Part model, mm, in its own coordinate system. Face numbers are marked on the shaded views. A direction names the side the tool comes from. Give positions to 0.01 mm unless a question says otherwise; leave off trailing zeros. Write each loop counter-clockwise with the first axis right and the second up, starting at its lowest first coordinate (ties: lowest second). Pieces come first, ordered by that corner, then holes. Notation, with made-up numbers: M 56,75 L 71,75 A15 ccw 71,100 Z; hole C 56,-8 d1. An arc over 180 degrees is marked long. Write item = value, one per line. Start each with the question number.
from build123d import *

# Parameters (mm, degrees)
SKETCH_1_W               = 38
SKETCH_1_H               = 11.5
EXTRUDE_1_DEPTH          = 1.6
EXTRUDE_START            = 1.6
SKETCH_1_3_W             = 38
SKETCH_1_3_H             = 1
SKETCH_1_3_W_2           = 1.5
SKETCH_1_3_H_2           = 11.5
EXTRUDE_2_DEPTH          = 1.5
EXTRUDE_START_2          = 3.1
EXTRUDE_3_DEPTH          = 8.4
SKETCH_2_4_W             = 2.4
SKETCH_2_4_H             = 1.5
EXTRUDE_5_DEPTH          = 3.1
CUT_EXTRUDE_1_DEPTH      = 22.744252114
FILLET_1_R               = 3
EXTRUDE_4_REACH          = 28.684
SKETCH_3_R               = 1.6
CUT_EXTRUDE_2_DEPTH      = 27.684499246
CUT_EXTRUDE_2_DEPTH_BACK = 27.684499246
SKETCH_3_3_R             = 1.7
SKETCH_3_3_W             = 6.5
SKETCH_3_3_H             = 1.7
SKETCH_3_3_W_2           = 3.4
SKETCH_3_3_H_2           = 3.1
FILLET_2_R               = 2.8
FILLET_3_R               = 2.5
FILLET_4_R               = 1
FILLET_5_R               = 0.5
FILLET_6_R               = 2


with BuildPart() as part:
    # 草图1 → 凸台-拉伸1 (new body)
    with BuildSketch(Plane(origin=(0, 0, 0), x_dir=(1, 0, 0), z_dir=(0, 1, 0))):
        Rectangle(SKETCH_1_W, SKETCH_1_H)
    extrude(amount=EXTRUDE_1_DEPTH)

    # 草图1<3> → 凸台-拉伸2 (add)
    with BuildSketch(Plane(origin=(0, 0, 0), x_dir=(1, 0, 0), z_dir=(0, 1, 0)).offset(EXTRUDE_START)):
        with Locations((0, 3.75)):
            Rectangle(SKETCH_1_3_W, SKETCH_1_3_H)
        Rectangle(SKETCH_1_3_W, SKETCH_1_3_H)
        with Locations((0, -3.75)):
            Rectangle(SKETCH_1_3_W, SKETCH_1_3_H)
        with Locations((-11.75, 0)):
            Rectangle(SKETCH_1_3_W_2, SKETCH_1_3_H_2)
        with Locations((11.75, 0)):
            Rectangle(SKETCH_1_3_W_2, SKETCH_1_3_H_2)
    extrude(amount=EXTRUDE_2_DEPTH)

    # 草图2 → 凸台-拉伸3 (add)
    with BuildSketch(Plane(origin=(0, 0, 0), x_dir=(1, 0, 0), z_dir=(0, 1, 0)).offset(EXTRUDE_START_2)):
        Polygon((-3.3, 9.05), (-5.1, 9.05), (-5.1, -2.15), (-7.5, -2.15), (-7.5, -9.15), (-5.5, -9.15), (-5.5, -2.55), (-3.3, -2.55), align=None)
        Polygon((5.1, 9.05), (3.3, 9.05), (3.3, -2.55), (5.5, -2.55), (5.5, -9.15), (7.5, -9.15), (7.5, -2.15), (5.1, -2.15), align=None)
    extrude(amount=-EXTRUDE_3_DEPTH)

    # 草图2<4> → 凸台-拉伸5 (add)
    with BuildSketch(Plane(origin=(0, 0, 0), x_dir=(1, 0, 0), z_dir=(0, 1, 0))):
        with Locations((-6.3, 5)):
            Rectangle(SKETCH_2_4_W, SKETCH_2_4_H)
        with Locations((6.3, 5)):
            Rectangle(SKETCH_2_4_W, SKETCH_2_4_H)
    extrude(amount=EXTRUDE_5_DEPTH)

    # 草图2<3> → 切除-拉伸1 (cut, through all)
    with BuildSketch(Plane(origin=(0, 0, 0), x_dir=(1, 0, 0), z_dir=(0, 1, 0))):
        Polygon((0, -9.15), (0, -2.55), (-3.3, -2.55), (-5.1, -2.55), (-5.5, -2.55), (-5.5, -9.15), align=None)
        Polygon((3.3, -2.55), (0, -2.55), (0, -9.15), (5.5, -9.15), (5.5, -2.55), (5.1, -2.55), align=None)
    extrude(amount=CUT_EXTRUDE_1_DEPTH, mode=Mode.SUBTRACT)

    # 圆角1
    # the kernel refuses this fillet: 3 mm, written as the material it adds along each edge
    with BuildSketch(Plane(origin=(5.1, 7.348469228, 2.15), x_dir=(0, 0, -1), z_dir=(0, -1, 0))) as fillet_1_piece_1_section:
        with BuildLine():
            CenterArc((2.939387691, 3), FILLET_1_R, 191.536959033, 78.463040967)
            Line((0, 2.4), (0, 0))
            Line((0, 0), (2.939387691, 0))
        make_face()
    fillet_1_piece_1 = extrude(amount=12.648469228, mode=Mode.PRIVATE)
    fillet_1_piece_1 = split(fillet_1_piece_1, bisect_by=Plane(origin=(5.102900281, 1.6, -0.644495887), z_dir=(0, -1, 0)), keep=Keep.TOP, mode=Mode.PRIVATE)
    add(fillet_1_piece_1)
    with BuildSketch(Plane(origin=(-5.1, 0, 2.15), x_dir=(0, 0, -1), z_dir=(0, -1, 0))) as fillet_1_piece_2:
        with BuildLine():
            CenterArc((2.939387691, -3), FILLET_1_R, 90, 78.463040967)
            Line((0, -2.4), (0, 0))
            Line((0, 0), (2.939387691, 0))
        make_face()
    extrude(amount=5.3)

    # 草图3 → 凸台-拉伸4 (add, up to next)
    with BuildSketch(Plane(origin=(-5.5, 0, 0), x_dir=(0, 0, -1), z_dir=(1, 0, 0)), mode=Mode.PRIVATE) as extrude_4_sk1:
        with Locations((-6.83, -2.5)):
            Circle(SKETCH_3_R)
    extrude_4_tool1 = extrude(extrude_4_sk1.sketch, amount=EXTRUDE_4_REACH, mode=Mode.PRIVATE) - part.part
    add(extrude_4_tool1.solids().sort_by_distance((-5.5, -2.5, 6.83))[0])

    # 草图3<3> → 切除-拉伸2 (cut, two sides: drawn at the far end of the back side and taken through both)
    with BuildSketch(Plane(origin=(-5.5, 0, 0), x_dir=(0, 0, -1), z_dir=(1, 0, 0)).offset(-CUT_EXTRUDE_2_DEPTH_BACK)):
        with Locations((5.75, -2.5)):
            Circle(SKETCH_3_3_R)
        with Locations((5.8, -4.45)):
            Rectangle(SKETCH_3_3_W, SKETCH_3_3_H)
        with Locations((-7.45, 1.55)):
            Rectangle(SKETCH_3_3_W_2, SKETCH_3_3_H_2)
    extrude(amount=CUT_EXTRUDE_2_DEPTH + CUT_EXTRUDE_2_DEPTH_BACK, mode=Mode.SUBTRACT)

    # 圆角2
    # the kernel refuses this fillet: 2.8 mm, written as the material it takes off along each edge
    with BuildSketch(Plane(origin=(-1.5, 0, 9.15), x_dir=(0, 0, -1), z_dir=(1, 0, 0)), Plane(origin=(-14.5, 0, 9.15), x_dir=(0, 0, -1), z_dir=(1, 0, 0))) as fillet_2_piece_1:
        with BuildLine():
            CenterArc((FILLET_2_R, -FILLET_2_R), FILLET_2_R, 90, 90)
            Line((0, -FILLET_2_R), (0, 0))
            Line((0, 0), (FILLET_2_R, 0))
        make_face()
    extrude(amount=16, mode=Mode.SUBTRACT)
    with BuildSketch(Plane(origin=(-1.5, -5.3, 9.15), x_dir=(0, 0, -1), z_dir=(1, 0, 0)), Plane(origin=(-14.5, -5.3, 9.15), x_dir=(0, 0, -1), z_dir=(1, 0, 0))) as fillet_2_piece_2:
        with BuildLine():
            CenterArc((FILLET_2_R, FILLET_2_R), FILLET_2_R, 180, 90)
            Line((0, FILLET_2_R), (0, 0))
            Line((0, 0), (FILLET_2_R, 0))
        make_face()
    extrude(amount=16, mode=Mode.SUBTRACT)

    # 圆角3
    fillet_3_edges = [part.edges().sort_by_distance(p)[0] for p in [
        (-4.2, 3.1, -9.05),
        (4.2, 3.1, -9.05),
    ]]
    fillet(fillet_3_edges, radius=FILLET_3_R)

    # 圆角4
    fillet_4_edges = [part.edges().sort_by_distance(p)[0] for p in [
        (-4.2, -3.6, -9.05),
        (4.2, -3.6, -9.05),
    ]]
    fillet(fillet_4_edges, radius=FILLET_4_R)

    # 圆角5
    fillet_5_edges = [part.edges().sort_by_distance(p)[0] for p in [
        (-4.2, -3.6, -4.45385186),
        (4.2, -3.6, -4.45385186),
        (-4.2, -3.6, -7.04614814),
        (4.2, -3.6, -7.04614814),
    ]]
    fillet(fillet_5_edges, radius=FILLET_5_R)

    # 圆角6
    # the kernel refuses this fillet: 2 mm, written as the material it adds along each edge
    with BuildSketch(Plane(origin=(5.1, 3.1, 2.15), x_dir=(0, 0, -1), z_dir=(0, -1, 0))) as fillet_6_piece_1:
        with BuildLine():
            CenterArc((2, 1.969136867), FILLET_6_R, 180, 79.921341892)
            Line((0, 1.969136867), (-0.04, 1.969136867))
            Line((-0.04, 1.969136867), (-0.04, 0))
            Line((-0.04, 0), (0, -0.04))
            ThreePointArc((0, -0.04), (0.825, -0.04), (1.643, -0.039382737))
            Line((1.643, -0.039382737), (1.65, 0))
        make_face()
    extrude(amount=6.422842167)
    with BuildSketch(Plane(origin=(-5.1, 3.1, 2.15), x_dir=(-1, 0, 0), z_dir=(0, -1, 0))) as fillet_6_piece_2:
        with BuildLine():
            CenterArc((1.969136867, 2), FILLET_6_R, 190.078658108, 79.921341892)
            Line((0, 1.65), (-0.039382737, 1.643))
            ThreePointArc((-0.039382737, 1.643), (-0.04, 0.825), (-0.04, 0))
            Line((-0.04, 0), (0, -0.04))
            Line((0, -0.04), (1.969136867, -0.04))
            Line((1.969136867, -0.04), (1.969136867, 0))
        make_face()
    extrude(amount=6.422842167)


solid = part.part
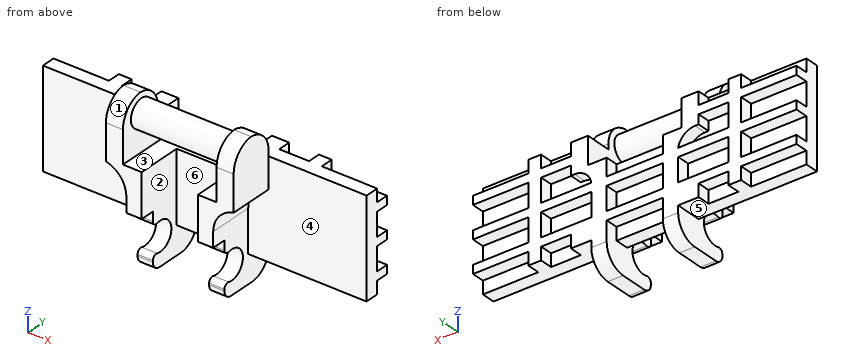
Q1. Tool access for the marked faces 4, 5 and 6: list every direction of +Z, -Z, +X, -X, +Y, -Y with a clear straight run to the whole face (end or side of a thin tool).
Q2. Slice it at C-C (z = -1.25). Give the cut face in (x, y).
Q3. Slice it at A-A (y = -1.75). Give the cut face in (x, z), and give its area (3 significant figures).
Q4. Two-plate mould, pull along X, no slides. Class the marked faces 1, 2 and 3: +X half, -X half, draft (parallel to the pull), parting line (faces both ways), or undercut.
Q5. Slice it at B-B (x = -10). Give the cut face in (y, z), and give its area (3 significant figures).
Q6. Probe line 1 along X through (y, z) = (2.25, -1.75); line 2 along Z through (x, y) = (-15.5, 2.25); line 3 along X through (y, z) = (-0.5, -4.75). List the from-to ranges inside material, lowest first.
Q7. Slice it at D-D (z = -5). Give the cut face in (x, y).
Q8. Drop flat-ended pins along their axis: P1, Ø1.6, axis at x = -8.5, y = 2, coming from the +Z side; P2, Ø0.5, axis at x = 7, y = 2.5, coming from the -Z side; P3, Ø1.2, axis at x = -8.5, z = 5, coming from the +Y side. Give the stop position or say it passes through.
Working result:
q1.face_4 = -Z, +X, -Y
q1.face_5 = -Z, -X, +Y, -Y
q1.face_6 = +Z, -Z, -Y
q2.outline = M -19,0 L -5.1,0 L -5.1,-5.3 L -3.3,-5.3 L -3.3,0 L 3.3,0 L 3.3,-5.3 L 5.1,-5.3 L 5.1,0 L 19,0 L 19,1.6 L 12.5,1.6 L 12.5,3.1 L 11,3.1 L 11,1.6 L 5.1,1.6 L 5.1,3.1 L 3.3,3.1 L 3.3,1.6 L -3.3,1.6 L -3.3,3.1 L -5.1,3.1 L -5.1,1.6 L -11,1.6 L -11,3.1 L -12.5,3.1 L -12.5,1.6 L -19,1.6 Z
q3.outline = M -7.5,2.15 A3 cw -5.1,-0.79 L -5.1,-4.22 L -3.3,-4.22 L -3.3,2.55 L -5.5,2.55 L -5.5,5.42 L 5.5,5.42 L 5.5,2.55 L 3.3,2.55 L 3.3,-4.22 L 5.1,-4.22 L 5.1,-0.79 A3 cw 7.5,2.15 L 7.5,8.95 L 5.5,8.95 L 5.5,8.24 L -5.5,8.24 L -5.5,8.95 L -7.5,8.95 Z; M -5.1,-9.05 L -3.3,-9.05 L -3.3,-7.28 L -5.1,-7.28 Z; M 3.3,-9.05 L 5.1,-9.05 L 5.1,-7.28 L 3.3,-7.28 Z
q3.area = 92.9 mm2
q4.face_1 = draft
q4.face_2 = undercut
q4.face_3 = undercut
q5.outline = M 0,-5.75 L 1.6,-5.75 L 1.6,-4.25 L 3.1,-4.25 L 3.1,-3.25 L 1.6,-3.25 L 1.6,-0.5 L 3.1,-0.5 L 3.1,0.5 L 1.6,0.5 L 1.6,3.25 L 3.1,3.25 L 3.1,4.25 L 1.6,4.25 L 1.6,5.75 L 0,5.75 Z
q5.area = 22.9 mm2
q6.line_1 = -12.5 to -11, -5.1 to -3.3, 3.3 to 5.1, 11 to 12.5
q6.line_2 = -4.25 to -3.25, -0.5 to 0.5, 3.25 to 4.25
q6.line_3 = -5.1 to -3.3, 3.3 to 5.1
q7.outline = M -19,0 L -5.1,0 L -5.1,-0.97 L -3.3,-0.97 L -3.3,0 L 3.3,0 L 3.3,-0.97 L 5.1,-0.97 L 5.1,0 L 19,0 L 19,1.6 L 12.5,1.6 L 12.5,3.1 L 11,3.1 L 11,1.6 L 7.5,1.6 L 7.5,3.1 L 3.3,3.1 L 3.3,1.6 L -3.3,1.6 L -3.3,3.1 L -7.5,3.1 L -7.5,1.6 L -11,1.6 L -11,3.1 L -12.5,3.1 L -12.5,1.6 L -19,1.6 Z
q8.P1 = 5.75
q8.P2 = -5.75
q8.P3 = 1.6
